Autodesk Inventor part; units mm, degrees
ref_plane "YZ Plane" through (0, 0, 0) normal (1, 0, 0) x (0, 1, 0)
ref_plane "XZ Plane" through (0, 0, 0) normal (0, 1, 0) x (-1, 0, 0)
ref_plane "XY Plane" through (0, 0, 0) normal (0, 0, 1) x (1, 0, 0)
sketch "Sketch1" plane through (0, 0, 0) normal (0, 1, 0) x (-1, 0, 0)
  line L0 (0, 0) -> (15, 0)
  line L1 (15, 0) -> (15, 12.5)
  line L2 (15, 12.5) -> (0, 12.5)
  line L3 (0, 12.5) -> (0, 0)
  dimension "d0" = 15
  dimension "d1" = 12.5
extrude "Extrusion1" add sketch "Sketch1" along normal blind 2
sketch "Sketch2" plane through (-15, 0, 12.5) normal (0, 0, 1) x (1, 0, 0)
  line L0 (0, 0) -> (15, 0)
  line L1 (15, 0) -> (15, 8.5)
  line L2 (15, 8.5) -> (0, 8.5)
  line L3 (0, 8.5) -> (0, 0)
  point P0 (15, 0)
  dimension "d4" = 8.5
  dimension "d5" = 15
extrude "Extrusion2" add sketch "Sketch2" along normal blind 1.5
sketch "Sketch3" plane through (0, 0, 0) normal (1, 0, 0) x (0, 0, -1)
  line L0 (-14, 8.5) -> (-14, 0)
  line L1 (-14, 8.5) -> (0, 8.5)
  line L2 (0, 8.5) -> (0, 0)
  line L3 (0, 0) -> (-14, 0)
  line L4 (-14, 0) -> (-14, 8.5)
  point P0 (-14, 0)
extrude "Extrusion3" add sketch "Sketch3" along normal blind 1.5
sketch "Sketch4" plane through (-15, 0, 12.5) normal (0, 0, -1) x (-1, 0, 0)
  line L0 (-15, 8.5) -> (0, 8.5)
  line L1 (-15, 2) -> (-15, 8.5)
  line L2 (0, 8.5) -> (-15, 8.5)
  line L3 (-15, 8.5) -> (-15, 7)
  line L4 (-15, 7) -> (0, 7)
  line L5 (0, 7) -> (0, 8.5)
  point P0 (-15, 0)
  dimension "d11" = 1.5
extrude "Extrusion4" add sketch "Sketch4" along normal blind 1
sketch "Sketch5" plane through (0, 2, 0) normal (0, 1, 0) x (1, 0, 0)
  circle A0 centre (-10, -6.25) radius 2.5
  line L0 (-15, 0) -> (-15, -12.5)
  line L1 (-15, -14) -> (1.5, -14)
  point P0 (0, 0)
  dimension "d14" = 5
  dimension "d15" = 5
  dimension "d28" = 7.75
extrude "Extrusion5" cut sketch "Sketch5" against normal blind 1.2
sketch "Sketch6" plane through (-10, 0.8, 6.25) normal (0, 1, 0) x (1, 0, 0)
  circle A0 centre (0, 0) radius 2.5
  circle A1 centre (0, 0) radius 1.5
  point P0 (10, 6.25)
  dimension "d29" = 3
extrude "Extrusion6" cut sketch "Sketch6" against normal blind 1.2 contours A1
sketch "Sketch7" plane through (-15, 0, 0) normal (0, 0, -1) x (-1, 0, 0)
  line L0 (-16.5, 0) -> (0, 0)
  line L1 (0, 0) -> (0, 2)
  line L2 (0, 2) -> (-16.5, 2)
  line L3 (-16.5, 2) -> (-16.5, 0)
  line L4 (-15, 8.5) -> (-16.5, 8.5)
  line L5 (-16.5, 2) -> (-15, 2)
  line L6 (-15, 2) -> (-15, 8.5)
  line L7 (-15, 8.5) -> (-16.5, 8.5)
  line L8 (-16.5, 8.5) -> (-16.5, 2)
  line L9 (0, 8.5) -> (-15, 8.5)
  line L10 (-15, 2) -> (0, 2)
  line L11 (0, 2) -> (0, 8.5)
  line L12 (0, 8.5) -> (-15, 8.5)
  line L13 (-15, 8.5) -> (-15, 2)
  point P0 (-15, 0)
extrude "Extrusion7" add sketch "Sketch7" along normal blind 1.5
sketch "Sketch8" plane through (-15, 0, 0) normal (0, 0, 1) x (1, 0, 0)
  line L0 (0, 8.5) -> (15, 8.5)
  line L1 (0, 8.5) -> (15, 8.5)
  line L2 (15, 8.5) -> (15, 7)
  line L3 (15, 7) -> (0, 7)
  line L4 (0, 7) -> (0, 8.5)
  point P0 (15, 0)
  dimension "d25" = 1.5
extrude "Extrusion8" add sketch "Sketch8" along normal blind 1
properties part number "LuftSensorHållare"
Here's how the part is built. I have some questions about the finished solid (model axes, mm). A direction names the side the tool comes from. Coordinates: 2 decimals unless noted, no trailing zeros. Loops run counter-clockwise (first coordinate to the right, second up) from the corner with the lowest first, then second, coordinate; pieces in that order, holes last. Notation, with made-up numbers: (-4, 19) -> (54, 19) arc R18 ccw to (54, 48) -> close; hole circle Ø8 at (17, 78.25). An arc over 180 degrees is marked (long way). Use one line per item in the form item = value. Start each with the question number.
(1) Will these pins go through, and if not, where does the flat tip stop? pin 1 (4 mm diameter, centred on x = -10, z = 6.25, fed in from +Y); pin 2 (6 mm diameter, centred on x = -9, z = 5.5, fed in from +Y); pin 3 (3 mm diameter, centred on y = 6, z = 7.5, fed in from -X).
(2) We'd pull the mould along Z, two halves only. Please class faces 4 (the face through (-7, 4, 14)), 5 (the face through (-5, 8.5, -1)), 6 (the face through (-7, 4, -1.5)), 7 (the face through (-7, 2, 6)): pulls with the +Z half, pulls with the -Z half, needs draft (parallel to the pull), parting line crosses it, or undercut.
(3) If we section it at A-A (x = -10): Please give me the cut outline in (y, z), then the cut area to 3 significant figures.
(4) On a 3-axis mill with a long thin cutter (end or side, diameter ignored), from which of +Z, -Z, +X, -X, +Y, -Y can I reach the whole of each face in a straight line? I mean faces 1 (the face through (-7.4, 7, 0.5)), 2 (the face through (-10, 0.8, 8)), 3 (the face through (-8, 8, 1)). Say none if no direction works.
(5) If we section it at C-C (z = 0.25): Please give me the cut outline in (x, y).
(6) If we section it at D-D (y = 5.5): Please give me the cut outline in (x, z), then the cut area to 4 significant figures.
(7) Please list where these lines run through material, in increasing order: line 1 along Z through (x, y) = (-7, 4.5); line 2 along X through (y, z) = (0.3, 6.25); line 3 along Z through (x, y) = (-8.5, 7.5).
(8) If we section it at B-B (z = 6.25): Please give me the cut outline in (x, y), then the cut area to 4 significant figures.
Verdict:
q1.pin_1 = 0.8
q1.pin_2 = 2
q1.pin_3 = 0
q2.face_4 = pulls with the +Z half
q2.face_5 = needs draft
q2.face_6 = pulls with the -Z half
q2.face_7 = undercut
q3.outline = (0, -1.5) -> (8.5, -1.5) -> (8.5, 1) -> (7, 1) -> (7, 0) -> (2, 0) -> (2, 3.75) -> (0.8, 3.75) -> (0.8, 4.75) -> (0, 4.75) -> close; (0, 7.75) -> (0.8, 7.75) -> (0.8, 8.75) -> (2, 8.75) -> (2, 12.5) -> (7, 12.5) -> (7, 11.5) -> (8.5, 11.5) -> (8.5, 14) -> (0, 14) -> close
q3.area = 45.1 mm²
q4.face_1 = -X
q4.face_2 = +Y
q4.face_3 = -X, +Y
q5.outline = (-15, 0) -> (1.5, 0) -> (1.5, 8.5) -> (-15, 8.5) -> (-15, 7) -> (0, 7) -> (0, 2) -> (-15, 2) -> close
q6.outline = (-15, -1.5) -> (1.5, -1.5) -> (1.5, 14) -> (-15, 14) -> (-15, 12.5) -> (0, 12.5) -> (0, 0) -> (-15, 0) -> close
q6.area = 68.25 mm²
q7.line_1 = -1.5 to 0, 12.5 to 14
q7.line_2 = -15 to -11.5, -8.5 to 1.5
q7.line_3 = -1.5 to 1, 11.5 to 14
q8.outline = (-15, 0) -> (-11.5, 0) -> (-11.5, 0.8) -> (-12.5, 0.8) -> (-12.5, 2) -> (-15, 2) -> close; (-8.5, 0) -> (1.5, 0) -> (1.5, 8.5) -> (0, 8.5) -> (0, 2) -> (-7.5, 2) -> (-7.5, 0.8) -> (-8.5, 0.8) -> close
q8.area = 34.35 mm²
